from build123d import *

# Parameters (mm, degrees)
SKETCH_1_W      = 30
SKETCH_1_H      = 20
EXTRUDE_1_DEPTH = 40
SKETCH_2_R      = 2
EXTRUDE_2_DEPTH = 5
SKETCH_3_RX     = 30
SKETCH_3_RY     = 5
EXTRUDE_3_DEPTH = 5
SKETCH_4_W      = 37.348500324
SKETCH_4_H      = 1
EXTRUDE_4_DEPTH = 2
EXTRUDE_START   = -2
EXTRUDE_5_DEPTH = 2
SKETCH_6_RX     = 29.994547564
SKETCH_6_RY     = 5.00002525
EXTRUDE_6_DEPTH = 5


# Read off the part's stored shape, not the designer's step: 凸台-拉伸5
with BuildPart() as part:
    # 草图1 → 凸台-拉伸1 (new body)
    with BuildSketch(Plane.XY):
        with Locations((15, 10)):
            Rectangle(SKETCH_1_W, SKETCH_1_H)
    extrude(amount=EXTRUDE_1_DEPTH)

    # 草图2 → 凸台-拉伸2 (add)
    with BuildSketch(Plane.ZY):
        with Locations(Location((30, 10, 0), (0, 0, 180))):
            Circle(SKETCH_2_R)
    extrude(amount=EXTRUDE_2_DEPTH)

    # 草图3 → 凸台-拉伸3 (add)
    with BuildSketch(Plane.ZY.offset(5)):
        with Locations(Location((30, 10), (0, 0, -103.92099691))):
            Ellipse(SKETCH_3_RX, SKETCH_3_RY)
    extrude(amount=EXTRUDE_3_DEPTH)

    # 草图4 → 凸台-拉伸4 (add)
    with BuildSketch(Plane.ZY.offset(10)):
        with Locations((18.674250162, 39.574648358)):
            Rectangle(SKETCH_4_W, SKETCH_4_H)
    extrude(amount=-EXTRUDE_4_DEPTH)

    # 凸台-拉伸5 outline → 凸台-拉伸5 (add)
    with BuildSketch(Plane.ZY.offset(10).offset(EXTRUDE_START)):
        with BuildLine():
            Line((39.862468471, -21), (39.619125683, 32.967296936))
            add(Edge.make_bspline(
                [(39.619125683, 32.967296936), (39.589392589, 39.561347803), (37.614649654, 40.050686248)],
                knots=[5.629361553, 5.629361553, 5.629361553, 6.283185307, 6.283185307, 6.283185307], degree=2, weights=[1, 0.947038516, 1]))
            Line((37.614649654, 40.050686248), (37.348500324, 40.050855796))
            Line((37.348500324, 40.050855796), (37.348500324, 39.074648358))
            add(Edge.make_bspline(
                [(38.697434301, 33.514015855), (38.694345199, 38.494694197), (37.348500324, 39.074648358)],
                knots=[5.657287765, 5.657287765, 5.657287765, 6.250122592, 6.250122592, 6.250122592], degree=2, weights=[0.790463711, 0.847402464, 0.984462923]))
            Line((38.697434301, 33.514015855), (38.765118588, -21))
            Line((38.765118588, -21), (39.862468471, -21))
        make_face()
    extrude(amount=EXTRUDE_5_DEPTH)

    # 草图6 → 凸台-拉伸6 (add)
    with BuildSketch(Plane.ZY.offset(10)):
        with Locations(Location((30, 10), (0, 0, -103.736326108))):
            Ellipse(SKETCH_6_RX, SKETCH_6_RY)
    extrude(amount=EXTRUDE_6_DEPTH)


solid = part.part
Design review of the part built by this model. Coordinates are the model's own, in mm. A direction names the side the tool comes from. Coordinates: 2 decimals unless noted, no trailing zeros. Order: outer loops, then holes, each group sorted by start corner. A loop starts at its lowest first (then second) coordinate and runs counter-clockwise, first axis right, second up. Notation, with made-up numbers: (37, 19) -> (52, 19) arc R15 cw to (52, 37) -> close; hole circle Ø3 at (14.25, 27.5). An arc over 180 degrees is marked (long way). One line per item, written item: value.
1) Draft analysis for pull direction X (two halves, no side actions). For faces 4 (the face through (-2.465, 9.399, 28.092)), 5 (the face through (-15, 10, 30)), 6 (the face through (-9, 40.075, 18)), 7 (the face through (-8, 23, 39)), state which applies: +X half, -X half, draft (parallel to the pull), parting line (faces both ways), or undercut.
Output values:
face 4: undercut
face 5: -X half
face 6: draft
face 7: undercut
2) We need section A-A, the plane z = 18.5. Give the boundary of the cut face in (x, y), then the cut area to 3 significant figures.
Output values:
outline: (-10, 39.07) -> (-8, 39.07) -> (-8, 40.07) -> (-10, 40.07) -> close; (0, 0) -> (30, 0) -> (30, 20) -> (0, 20) -> close
area: 602 mm2
3) We need section C-C, the plane z = 24. Count the separate pieces of the cut face and the enclosed holes in it, then the cut area to 3 significant figures.
Output values:
separate pieces: 3
enclosed holes: 0
area: 852 mm2
4) Clearance check with flat-ended pins moving along their axes: P1, Ø6, axis at x = -9.5, y = 18, coming from the -Z side; P2, Ø16, axis at y = 15, z = 12, coming from the -X side; P3, Ø1.6, axis at x = -8.5, z = 24.5, coming from the -Y side; P4, Ø6, axis at x = -3.5, z = 12.5, coming from the +Y side. State where each tip first meets the part, or that it passes through.
Output values:
P1: stops at z = 26.13
P2: stops at x = 0
P3: stops at y = -18.91
P4: passes through
5) To check wall thickness, follow probe 1 along X at (y, z) = (14.5, 35); probe 2 along X at (y, z) = (20.5, 35.5); probe 3 along Y at (x, z) = (15, 34.5). State the ranges of each line that lie inside material, in increasing order. Write a range as [from, to].
Output values:
probe 1: x = [-15, -5], [0, 30]
probe 2: x = [-15, -5]
probe 3: y = [0, 20]
6) Machinability: for faces 1 (the face through (15, 20, 20)), 2 (the face through (15, 0, 20)), 3 (the face through (30, 10, 20)), which of the approach directions +Z, -Z, +X, -X, +Y, -Y give a long, thin tool a straight path to every point of the face, cutting with its end or side? Answer none if there is none.
Output values:
face 1: +Z, -Z, +X, +Y
face 2: +Z, -Z, +X, -Y
face 3: +Z, -Z, +X, +Y, -Y
7) We need section B-B, the plane x = 11.5. Give the boundary of the cut face in (y, z).
Output values:
outline: (0, 0) -> (20, 0) -> (20, 40) -> (0, 40) -> close
